Can you work these out from the model? Positions are in its coordinate system, mm. A direction names the side the tool comes from. Round coordinates to 2 decimals unless told otherwise and drop trailing zeros. Write each loop counter-clockwise with the first axis right and the second up, starting at its lowest first coordinate (ties: lowest second). Pieces come first, ordered by that corner, then holes. Notation, with made-up numbers: (51, 61.5) -> (102, 61.5) arc R16 ccw to (102, 88.5) -> close; hole circle Ø5 at (63, 49.5). An arc over 180 degrees is marked (long way). Use CSV: the item, a comma, the result in double quotes.
```python
from build123d import *

# Parameters (mm, degrees)
F0_R          = 12.7
F1_DEPTH      = 330.2
F1_DEPTH_BACK = 25.4
F3_R          = 19.05
F4_DEPTH      = 25.4
F5_R          = 12.7
F6_DEPTH      = 25.4
F6_DEPTH_BACK = 25.4
F7_R          = 6.35
F8_DEPTH      = 25.401
F8_DEPTH_BACK = 25.401


with BuildPart() as f1:
    # F0 (on Top) → F1 (new body, two sides)
    with BuildSketch(Plane.XY) as f1_sk:
        Circle(F0_R)
    extrude(amount=-F1_DEPTH)
    extrude(f1_sk.sketch, amount=F1_DEPTH_BACK)

    # F3 (on offset) → F4 (join)
    with BuildSketch(Plane.XY.offset(-203.2)):
        Circle(F3_R)
    extrude(amount=-F4_DEPTH)

    # F5 (on Front) → F6 (join, two sides)
    with BuildSketch(Plane.XZ) as f6_sk:
        with Locations((0, 25.4)):
            Circle(F5_R)
    extrude(amount=F6_DEPTH)
    extrude(f6_sk.sketch, amount=-F6_DEPTH_BACK)

    # F7 (on Front) → F8 (cut, two sides)
    with BuildSketch(Plane.XZ) as f8_sk:
        with Locations((0, 25.4)):
            Circle(F7_R)
    extrude(amount=-F8_DEPTH, mode=Mode.SUBTRACT)
    extrude(f8_sk.sketch, amount=F8_DEPTH_BACK, mode=Mode.SUBTRACT)


solid = f1.part
```
Q1. Suppose I cut it at A-A (x = 0). Write out the boundary of the cut face in (y, z).
Resolved:
outline,"(-25.4, 12.7) -> (-12.7, 12.7) -> (-12.7, -203.2) -> (-19.05, -203.2) -> (-19.05, -228.6) -> (-12.7, -228.6) -> (-12.7, -330.2) -> (12.7, -330.2) -> (12.7, -228.6) -> (19.05, -228.6) -> (19.05, -203.2) -> (12.7, -203.2) -> (12.7, 12.7) -> (25.4, 12.7) -> (25.4, 19.05) -> (-25.4, 19.05) -> close; (-25.4, 31.75) -> (25.4, 31.75) -> (25.4, 38.1) -> (-25.4, 38.1) -> close"
Q2. Suppose I cut it at B-B (y = 16). Write out the boundary of the cut face in (x, z), and give its area (3 significant figures).
Resolved:
outline,"circle Ø25.4 at (0, 25.4); (-10.34, -228.6) -> (10.34, -228.6) -> (10.34, -203.2) -> (-10.34, -203.2) -> close; hole circle Ø12.7 at (0, 25.4)"
area,"905 mm^2"
Q3. Suppose I cut it at D-D (y = -9). Write out the boundary of the cut face in (x, z), and give its area (3 significant figures).
Resolved:
outline,"(-16.79, -228.6) -> (-8.96, -228.6) -> (-8.96, -330.2) -> (8.96, -330.2) -> (8.96, -228.6) -> (16.79, -228.6) -> (16.79, -203.2) -> (8.96, -203.2) -> (8.96, 16.4) arc R12.7 ccw (long way) to (-8.96, 16.4) -> (-8.96, -203.2) -> (-16.79, -203.2) -> close; hole circle Ø12.7 at (0, 25.4)"
area,"6,940 mm^2"
Q4. On a 3-axis mill with a long thin cutter (end or side, diameter ignored), from which of +Z, -Z, +X, -X, +Y, -Y can I reach the whole of each face in a straight line? I mean faces 4 (the face through (4, -12.4, -203.2)), 5 (the face through (0, 0, -330.2)), 6 (the face through (-15.12, -11.59, -215.72)). Say none if no direction works.
Resolved:
face 4,"none"
face 5,"-Z, +X, -X, +Y, -Y"
face 6,"-Z"
Q5. Suppose I cut it at C-C (z = -6). Write out the boundary of the cut face in (x, y).
Resolved:
outline,"circle Ø25.4 at (0, 0)"
Q6. Will these pins go through, and if not, where does the flat tip stop? P1, Ø10, axis at x = -12, y = 7, coming from the +Z side; P2, Ø1, axis at x = 5, z = -199, coming from the +Y side; P3, Ø10, axis at x = 2, z = -39.5, coming from the +Y side; P4, Ø20.5, axis at x = 0, z = 25.4, coming from the +Y side.
Resolved:
P1,"stops at z = 36"
P2,"stops at y = 11.88"
P3,"stops at y = 12.7"
P4,"stops at y = 25.4"
Q7. If we mould it in two halves opening along Z, with no side actions, what happens to faces 1 (the face through (4, -12.4, -228.6)), 2 (the face through (-1.653, 12.592, -87.3)), 3 (the face through (-2.75, -12.4, -278.69))? For each: released by +Z, released by -Z, zero draft, split by the parting line, or undercut.
Resolved:
face 1,"released by -Z"
face 2,"undercut"
face 3,"zero draft"
Q8. Please list where these lines run through material, in increasing order: probe 1 along Z at (x, y) = (0, -11.5); probe 2 along X at (y, z) = (-7, 25); probe 3 along Z at (x, y) = (7, 11).
Resolved:
probe 1,"z = -330.2 to 19.05, 31.75 to 38.1"
probe 2,"x = -12.69 to -6.34, 6.34 to 12.69"
probe 3,"z = -228.6 to -203.2, 14.8 to 36"
